from build123d import *

# Parameters (mm, degrees)
SKETCH1_R                    = 70
BOSS_EXTRUDE1_DEPTH          = 12
TAP_DRILL_FOR_M12X1_5_TAP1_D = 10.5
CIRPATTERN1_COUNT            = 4


with BuildPart() as part:
    # Sketch1 → Boss-Extrude1 (new body)
    with BuildSketch(Plane.XY):
        Circle(SKETCH1_R)
    extrude(amount=BOSS_EXTRUDE1_DEPTH)

    # Tap Drill for M12x1.5 Tap1 (through all)
    with Locations(Plane(origin=(0, 50, 12), x_dir=(1, 0, 0), z_dir=(0, 0, 1))):
        with Locations((0, 0)):
            tap_drill_for_m12x1_5_tap1 = Hole(TAP_DRILL_FOR_M12X1_5_TAP1_D / 2)

    # CirPattern1: Tap Drill for M12x1.5 Tap1 ×4 about axis
    cirpattern1_axis = Axis((0, 0, 0), (0, 0, 1))
    for i in range(1, CIRPATTERN1_COUNT):
        add(tap_drill_for_m12x1_5_tap1.rotate(cirpattern1_axis, i * 360 / CIRPATTERN1_COUNT), mode=Mode.SUBTRACT)


solid = part.part
Part model, mm, in its own coordinate system. Coordinates: 2 decimals unless noted, no trailing zeros. Write each loop counter-clockwise with the first axis right and the second up, starting at its lowest first coordinate (ties: lowest second). Pieces come first, ordered by that corner, then holes. Notation, with made-up numbers: (61, 76) - (84, 76) arc R27 cw to (84, 100) - close; hole circle Ø3 at (43.25, -3.75). An arc over 180 degrees is marked (long way). Put each result on its own line as item: value.
1. Flat gauge pins, fed straight in: pin 1 Ø6 at (y, z) = (-20, 6.5) entering from -X; pin 2 Ø8.5 at (x, y) = (50, 0) entering from +Z; pin 3 Ø3 at (x, z) = (52.5, 8) entering from +Y; pin 4 Ø4 at (y, z) = (-39, 8) entering from -X. Where does each tip first touch, or does it go through?
Final values:
pin 1: stops at x = -67.9
pin 2: passes through
pin 3: stops at y = 47.95
pin 4: stops at x = -59.42
2. Two-plate mould, pull along Y, no slides. Class faces 1 (the cylindrical face through (-55.55, -42.594, 5.916)), 2 (the cylindrical face through (-0.683, -55.205, 5.916)), 3 (the cylindrical face through (-55.205, 0.683, 5.916)), 4 (the flat face through (-1, 1, 12)): +Y half, -Y half, draft (parallel to the pull), parting line (faces both ways), or undercut.
Final values:
face 1: parting line
face 2: undercut
face 3: undercut
face 4: draft
3. Band-saw the part on C-C (z = 4.5). Write the cut outline in (x, y), then the cut area to 3 significant figures.
Final values:
outline: circle Ø140 at (0, 0); hole circle Ø10.5 at (-50, 0); hole circle Ø10.5 at (0, -50); hole circle Ø10.5 at (0, 50); hole circle Ø10.5 at (50, 0)
area: 15,000 mm²
4. Band-saw the part on A-A (x = 0). Write the cut outline in (y, z).
Final values:
outline: (-70, 0) - (-55.25, 0) - (-55.25, 12) - (-70, 12) - close; (-44.75, 0) - (44.75, 0) - (44.75, 12) - (-44.75, 12) - close; (55.25, 0) - (70, 0) - (70, 12) - (55.25, 12) - close
5. Probe line 1 along Y through (x, z) = (0, 4.5); line 2 along X through (y, z) = (3.5, 5); line 3 along Y through (x, z) = (-50, 6.75). List the from-to ranges inside material, lowest first. Write a range as [from, to].
Final values:
line 1: y = [-70, -55.25], [-44.75, 44.75], [55.25, 70]
line 2: x = [-69.91, -53.91], [-46.09, 46.09], [53.91, 69.91]
line 3: y = [-48.99, -5.25], [5.25, 48.99]
6. Band-saw the part on D-D (x = -50). Write the cut outline in (y, z), then the cut area to 3 significant figures.
Final values:
outline: (-48.99, 0) - (-5.25, 0) - (-5.25, 12) - (-48.99, 12) - close; (5.25, 0) - (48.99, 0) - (48.99, 12) - (5.25, 12) - close
area: 1,050 mm²
